```python
from build123d import *

# Parameters (mm, degrees)
CROQUIS1_R              = 2.5
CROQUIS1_R_2            = 2
CROQUIS1_R_3            = 1.5
CROQUIS1_W              = 13
CROQUIS1_H              = 23
CROQUIS1_W_2            = 15
CROQUIS1_H_2            = 15
SALIENTE_EXTRUIR1_DEPTH = 3
CROQUIS2_W              = 20
CROQUIS2_H              = 72.999
CORTAR_EXTRUIR1_DEPTH   = 10
CROQUIS3_W              = 35
CROQUIS3_H              = 15
CORTAR_EXTRUIR2_DEPTH   = 10
CROQUIS4_R              = 1.5
CORTAR_EXTRUIR3_DEPTH   = 10
CORTAR_EXTRUIR4_DEPTH   = 10


with BuildPart() as part:
    # Croquis1 → Saliente-Extruir1 (new body)
    with BuildSketch(Plane(origin=(0, 0, 0), x_dir=(1, 0, 0), z_dir=(0, 1, 0))):
        with BuildLine():
            Line((0, 0), (-160, 0))
            Line((-160, 0), (-160, -70))
            ThreePointArc((-160, -70), (-154.142135624, -84.142135624), (-140, -90))
            Line((-140, -90), (-137, -90))
            Line((-137, -90), (-137, -89.999))
            Line((-137, -89.999), (-23, -89.999))
            Line((-23, -89.999), (-23, -90))
            Line((-23, -90), (-20, -90))
            ThreePointArc((-20, -90), (-5.857864376, -84.142135624), (0, -70))
            Line((0, -70), (0, 0))
        make_face()
        with Locations(Location((-101.245, -7, 0), (0, 0, 270))):
            Circle(CROQUIS1_R, mode=Mode.SUBTRACT)
        with Locations(Location((-58.755, -7, 0), (0, 0, 270))):
            Circle(CROQUIS1_R, mode=Mode.SUBTRACT)
        with Locations(Location((-27.5, -60, 0), (0, 0, 270))):
            Circle(CROQUIS1_R_2, mode=Mode.SUBTRACT)
        with Locations(Location((-52.5, -60, 0), (0, 0, 270))):
            Circle(CROQUIS1_R_2, mode=Mode.SUBTRACT)
        with Locations(Location((-27.5, -34, 0), (0, 0, 270))):
            Circle(CROQUIS1_R_2, mode=Mode.SUBTRACT)
        with Locations(Location((-52.5, -34, 0), (0, 0, 270))):
            Circle(CROQUIS1_R_2, mode=Mode.SUBTRACT)
        with Locations(Location((-107.5, -34, 0), (0, 0, 270))):
            Circle(CROQUIS1_R_2, mode=Mode.SUBTRACT)
        with Locations(Location((-132.5, -34, 0), (0, 0, 270))):
            Circle(CROQUIS1_R_2, mode=Mode.SUBTRACT)
        with Locations(Location((-132.5, -60, 0), (0, 0, 270))):
            Circle(CROQUIS1_R_2, mode=Mode.SUBTRACT)
        with Locations(Location((-107.5, -60, 0), (0, 0, 270))):
            Circle(CROQUIS1_R_2, mode=Mode.SUBTRACT)
        with Locations(Location((-80, -22.054, 0), (0, 0, 270))):
            Circle(CROQUIS1_R_3, mode=Mode.SUBTRACT)
        with Locations(Location((-80, -50.344, 0), (0, 0, 270))):
            Circle(CROQUIS1_R_3, mode=Mode.SUBTRACT)
        with Locations((-80, -36.199)):
            Rectangle(CROQUIS1_W, CROQUIS1_H, mode=Mode.SUBTRACT)
        with Locations((-97.5, -72.499)):
            Rectangle(CROQUIS1_W_2, CROQUIS1_H_2, mode=Mode.SUBTRACT)
        with Locations((-62.5, -72.499)):
            Rectangle(CROQUIS1_W_2, CROQUIS1_H_2, mode=Mode.SUBTRACT)
    extrude(amount=SALIENTE_EXTRUIR1_DEPTH)

    # Croquis2 → Cortar-Extruir1 (cut)
    with BuildSketch(Plane(origin=(0, 3, 0), x_dir=(1, 0, 0), z_dir=(0, 1, 0))):
        with Locations((-150, -46.4995)):
            Rectangle(CROQUIS2_W, CROQUIS2_H)
        with Locations((-10, -46.4995)):
            Rectangle(CROQUIS2_W, CROQUIS2_H)
    extrude(amount=-CORTAR_EXTRUIR1_DEPTH, mode=Mode.SUBTRACT)

    # Croquis3 → Cortar-Extruir2 (cut)
    with BuildSketch(Plane.XZ):
        with Locations((-80, 7.5)):
            Rectangle(CROQUIS3_W, CROQUIS3_H)
    extrude(amount=-CORTAR_EXTRUIR2_DEPTH, mode=Mode.SUBTRACT)

    # Croquis4 → Cortar-Extruir3 (cut)
    with BuildSketch(Plane(origin=(0, 0, 0), x_dir=(-1, 0, 0), z_dir=(0, -1, 0))):
        with Locations(Location((157, -7, 0), (0, 0, 90))):
            Circle(CROQUIS4_R)
        with Locations(Location((3, -7, 0), (0, 0, 90))):
            Circle(CROQUIS4_R)
        with Locations(Location((30, -86.999, 0), (0, 0, 90))):
            Circle(CROQUIS4_R)
        with Locations(Location((50, -86.999, 0), (0, 0, 90))):
            Circle(CROQUIS4_R)
        with Locations(Location((70, -86.999, 0), (0, 0, 90))):
            Circle(CROQUIS4_R)
        with Locations(Location((130, -86.999, 0), (0, 0, 90))):
            Circle(CROQUIS4_R)
        with Locations(Location((90, -86.999, 0), (0, 0, 90))):
            Circle(CROQUIS4_R)
        with Locations(Location((110, -86.999, 0), (0, 0, 90))):
            Circle(CROQUIS4_R)
        with Locations(Location((142.5, -86.999, 0), (0, 0, 90))):
            Circle(CROQUIS4_R)
        with Locations(Location((17.5, -86.999, 0), (0, 0, 90))):
            Circle(CROQUIS4_R)
    extrude(amount=-CORTAR_EXTRUIR3_DEPTH, mode=Mode.SUBTRACT)

    # Croquis5 → Cortar-Extruir4 (cut)
    with BuildSketch(Plane(origin=(0, 0, 0), x_dir=(-1, 0, 0), z_dir=(0, -1, 0))):
        with BuildLine():
            Line((98, -50), (94, -50))
            ThreePointArc((94, -50), (91.171572875, -48.828427125), (90, -46))
            Line((90, -46), (90, -24))
            ThreePointArc((90, -24), (91.171572875, -21.171572875), (94, -20))
            Line((94, -20), (98, -20))
            ThreePointArc((98, -20), (100.828427125, -21.171572875), (102, -24))
            Line((102, -24), (102, -46))
            ThreePointArc((102, -46), (100.828427125, -48.828427125), (98, -50))
        make_face()
        with BuildLine():
            Line((66.613773368, -50), (61.386226632, -50))
            ThreePointArc((61.386226632, -50), (58.991802818, -49.008197182), (58, -46.613773368))
            Line((58, -46.613773368), (58, -23.386226632))
            ThreePointArc((58, -23.386226632), (58.991802818, -20.991802818), (61.386226632, -20))
            Line((61.386226632, -20), (66.613773368, -20))
            ThreePointArc((66.613773368, -20), (69.008197182, -20.991802818), (70, -23.386226632))
            Line((70, -23.386226632), (70, -46.613773368))
            ThreePointArc((70, -46.613773368), (69.008197182, -49.008197182), (66.613773368, -50))
        make_face()
    extrude(amount=-CORTAR_EXTRUIR4_DEPTH, mode=Mode.SUBTRACT)


solid = part.part
```
The listing builds one solid part. Answer for the finished solid, in the listing's coordinates (mm). A direction names the side the tool comes from. Round coordinates to 2 decimals unless told otherwise and drop trailing zeros. Loops run counter-clockwise (first coordinate to the right, second up) from the corner with the lowest first, then second, coordinate; pieces in that order, holes last. Notation, with made-up numbers: (-26, 69) - (13, 69) arc R29 ccw to (13, 96) - close; hole circle Ø11 at (23, 28). An arc over 180 degrees is marked (long way). Return JSON: item names as keys, results as strings. Group by question number.
1. The part is cut by section D-D on y = 1.35. State how many separate pieces and enclosed holes the cut face has, then the cut area to 3 significant figures.
2. The part is cut by section C-C on x = -3. Determine the outline of the cut face in (y, z).
3. Consider probe 1 along Z at (x, y) = (-95, 0.2); probe 2 along X at (y, z) = (1.6, 7) (3 decimals); probe 3 along X at (y, z) = (0.9, 70). Determine where each line is inside the solid, lowest interval first.
4. The part is cut by section A-A on x = -64.5. Determine the outline of the cut face in (y, z).
5. Each of these flat-tipped pins is pushed along its axis until it touches: P1, Ø0.9, axis at y = 1.5, z = 31.5, coming from the +X side; P2, Ø10, axis at x = -24, z = 28, coming from the -Y side; P3, Ø1.5, axis at x = -6.5, y = 2, coming from the +Z side; P4, Ø0.9, axis at x = -81.5, y = 2, coming from the -Z side. Where does it stop, or does it pass through?
6. The mould has two halves that part along Z. Classify faces 5 (the flat face through (-81, 1, 89.999)), 6 (the cylindrical face through (-141.235, 1.479, 86.193)), 7 (the cylindrical face through (-29.274, 1.479, 34.923)), 8 (the flat face through (0, 1, 5)): pulls with the +Z half, pulls with the -Z half, needs draft (parallel to the pull), parting line crosses it, or undercut.
7. The part is cut by section B-B on z = 68. Determine the outline of the cut face in (x, y).
8. Which of the six approach directions +Z, -Z, +X, -X, +Y, -Y give full straight-line access (tool end or side, diameter ignored) to faces 1 (the flat face through (-62.5, 1, 7)), 2 (the flat face through (-98, 1, 64.999)), 3 (the flat face through (-148, 2, 82.999)), 4 (the flat face through (-20, 2, 47))?
Resolved:
{
 "1": {"separate pieces": "1", "enclosed holes": "27", "area": "9,150 mm²"},
 "2": {"outline": "(0, 0) - (3, 0) - (3, 5.5) - (0, 5.5) - close; (0, 8.5) - (3, 8.5) - (3, 10) - (0, 10) - close"},
 "3": {"probe 1": "z = 15 to 20, 50 to 65, 80 to 90", "probe 2": "x = -160 to -158.5, -155.5 to -103.745, -98.745 to -97.5, -62.5 to -61.255, -56.255 to -4.5, -1.5 to 0", "probe 3": "x = -140 to -105, -90 to -70, -55 to -20"},
 "4": {"outline": "(0, 15) - (3, 15) - (3, 20) - (0, 20) - close; (0, 50) - (3, 50) - (3, 65) - (0, 65) - close; (0, 80) - (3, 80) - (3, 90) - (0, 90) - close"},
 "5": {"P1": "stops at x = -20", "P2": "stops at y = 0", "P3": "stops at z = 85.41", "P4": "stops at z = 15"},
 "6": {"face 5": "pulls with the +Z half", "face 6": "undercut", "face 7": "undercut", "face 8": "needs draft"},
 "7": {"outline": "(-140, 0) - (-105, 0) - (-105, 3) - (-140, 3) - close; (-90, 0) - (-70, 0) - (-70, 3) - (-90, 3) - close; (-55, 0) - (-20, 0) - (-20, 3) - (-55, 3) - close"},
 "8": {"face 1": "-Z, +Y, -Y", "face 2": "+Y, -Y", "face 3": "-X, +Y, -Y", "face 4": "+X, +Y, -Y"}
}
